The listing builds one solid part. Answer for the finished solid, in the listing's coordinates (mm). A direction names the side the tool comes from. Give positions to 0.01 mm unless a question says otherwise; leave off trailing zeros. Loops run counter-clockwise (first coordinate to the right, second up) from the corner with the lowest first, then second, coordinate; pieces in that order, holes last. Notation, with made-up numbers: (66, 43) -> (74, 43) arc R25 ccw to (74, 58) -> close; hole circle Ø6 at (-1, 2.25). An arc over 180 degrees is marked (long way). One line per question, with ' | ' between items. Start each with the question number.
Autodesk Inventor part; units mm, degrees
ref_plane "YZ Plane" through (0, 0, 0) normal (1, 0, 0) x (0, 1, 0)
ref_plane "XZ Plane" through (0, 0, 0) normal (0, 1, 0) x (-1, 0, 0)
ref_plane "XY Plane" through (0, 0, 0) normal (0, 0, 1) x (1, 0, 0)
sketch "スケッチ1" plane through (0, 0, 0) normal (0, 0, 1) x (1, 0, 0)
  line L0 (-7.5, 7.5) -> (7.5, 7.5)
  line L1 (7.5, 7.5) -> (7.5, -7.5)
  line L2 (7.5, -7.5) -> (-7.5, -7.5)
  line L3 (-7.5, -7.5) -> (-7.5, 7.5)
  line L4 (-7.5, 7.5) -> (7.5, -7.5) construction
  line L5 (7.5, 7.5) -> (-7.5, -7.5) construction
  line L6 (-6.5, -6.5) -> (6.5, -6.5)
  line L7 (6.5, -6.5) -> (6.5, 6.5)
  line L8 (6.5, 6.5) -> (-6.5, 6.5)
  line L9 (-6.5, 6.5) -> (-6.5, -6.5)
  point P0 (0, 0)
  dimension "d0" = 15
  dimension "d1" = 15
extrude "押し出し1" add sketch "スケッチ1" along normal mid plane 300
sketch "スケッチ2" plane through (-7.5, -7.5, 150) normal (0, -1, 0) x (1, 0, 0)
  line L0 (7.5, -270) -> (7.5, -30)
  point P0 (7.5, -150)
  point P1 (7.5, -150)
  dimension "d4" = 240
hole "穴1" at (0, -7.5, 120) at (0, -7.5, -120) direction (0, 1, 0) diameter 3.2 end through all
sketch "スケッチ3" plane through (-7.5, -7.5, 150) normal (-1, 0, 0) x (0, 0, 1)
  line L0 (-285, 7.5) -> (-15, 7.5)
  point P0 (-150, 7.5)
  point P1 (-150, 7.5)
  dimension "d12" = 270
hole "穴2" at (-7.5, 0, -135) at (-7.5, 0, 135) direction (1, 0, 0) diameter 3.2 end through all
properties part number "回路角柱"
1. Straight lines are drawn through the part: L1, parallel to Z at x = 0, y = 7; L2, parallel to Z at x = 6.9, y = 0; L3, parallel to Y at x = -6.95, z = 135. For each, find the intervals that lie inside material, in ascending order.
2. Determine the mould class of faces 1 (the flat face through (0, -7.5, -2)), 2 (the flat face through (-7, 0, 150)), 3 (the flat face through (0, -6.5, -2)), 4 (the flat face through (0, 7.5, -2)) for opening direction Y: released by +Y, released by -Y, zero draft, split by the parting line, or undercut.
3. Each of these flat-tipped pins is pushed along its axis until it touches: pin 1 Ø4 at (x, z) = (0, -120) entering from +Y; pin 2 Ø2.5 at (x, z) = (0, -120) entering from +Y. Where does it stop, or does it pass through?
4. For faces 5 (the flat face through (-7, 0, -150)), 6 (the flat face through (6.5, 0, -2)), determine the directions among +Z, -Z, +X, -X, +Y, -Y from which every point of the face is accessible in a straight line to the end or side of a thin tool.
5. The part is cut by section A-A (z = -58.5). Write down the section's boundary in (x, y), plus the area to 3 significant figures.
Check sheet entries:
1) L1: z = -150 to -121.6, -118.4 to 118.4, 121.6 to 150 | L2: z = -150 to -136.6, -133.4 to 133.4, 136.6 to 150 | L3: y = -7.5 to -1.6, 1.6 to 7.5
2) face 1: released by -Y | face 2: zero draft | face 3: undercut | face 4: released by +Y
3) pin 1: stops at y = 7.5 | pin 2: passes through
4) face 5: -Z, +X, -X, +Y, -Y | face 6: +Z, -Z
5) outline: (-7.5, -7.5) -> (7.5, -7.5) -> (7.5, 7.5) -> (-7.5, 7.5) -> close; hole (-6.5, -6.5) -> (6.5, -6.5) -> (6.5, 6.5) -> (-6.5, 6.5) -> close | area: 56.0 mm^2
